```python
from build123d import *

# Parameters (mm, degrees)
SKETCH1_W           = 100
SKETCH1_H           = 100
BOSS_EXTRUDE1_DEPTH = 5.08
SKETCH2_R           = 40
BOSS_EXTRUDE2_DEPTH = 63.5
CHAMFER1_SIZE       = 5.08


with BuildPart() as part:
    # Sketch1 → Boss-Extrude1 (new body)
    with BuildSketch(Plane.XY):
        Rectangle(SKETCH1_W, SKETCH1_H)
    extrude(amount=BOSS_EXTRUDE1_DEPTH)

    # Sketch2 → Boss-Extrude2 (add)
    with BuildSketch(Plane.XY):
        Circle(SKETCH2_R)
    extrude(amount=BOSS_EXTRUDE2_DEPTH)

    # Chamfer1
    chamfer1_edges = [part.edges().sort_by_distance(p)[0] for p in [
        (-40, 0, 63.5),
    ]]
    chamfer(chamfer1_edges, length=CHAMFER1_SIZE)


solid = part.part
```
Could you check a few things on this model? Use its own coordinates, in mm. A direction names the side the tool comes from. Coordinates: 2 decimals unless noted, no trailing zeros. Loops run counter-clockwise (first coordinate to the right, second up) from the corner with the lowest first, then second, coordinate; pieces in that order, holes last.
1) Please list where these lines run through material, in increasing order: line 1 along Z through (x, y) = (41, -13); line 2 along X through (y, z) = (-16, 11.5); line 3 along X through (y, z) = (-18, 8).
Reported:
line 1: z = 0 to 5.08
line 2: x = -36.66 to 36.66
line 3: x = -35.72 to 35.72
2) Thinking about a two-plate mould opening in X: for faces 3 (the face through (33.543, 10.563, 63.253)), 4 (the face through (-1, -50, 3)), 5 (the face through (-50, -1, 3)), which applies, released by +X, released by -X, zero draft, split by the parting line, or undercut?
Reported:
face 3: split by the parting line
face 4: zero draft
face 5: released by -X
3) Imagine slicing it at C-C (z = 18.5). List the corners of the cut face in (x, y) for me, and give its area (3 significant figures).
Reported:
outline: circle Ø80 at (0, 0)
area: 5,030 mm2
4) Which directions (+Z, -Z, +X, -X, +Y, -Y) give clear straight access to the entire face, cutting with the end or side of a thin tool? Please do faces 1 (the face through (-1, 1, 0)), 2 (the face through (-34, 23, 5.08)).
Reported:
face 1: -Z, +X, -X, +Y, -Y
face 2: +Z
5) Imagine slicing it at A-A (y = 0). List the corners of the cut face in (x, z) for me, and give its area (3 significant figures).
Reported:
outline: (-50, 0) - (50, 0) - (50, 5.08) - (40, 5.08) - (40, 58.42) - (34.92, 63.5) - (-34.92, 63.5) - (-40, 58.42) - (-40, 5.08) - (-50, 5.08) - close
area: 5,160 mm2
6) Will these pins go through, and if not, where does the flat tip stop? pin 1 Ø3 at (x, z) = (-16, 40) entering from -Y; pin 2 Ø6 at (y, z) = (-21, 20) entering from -X; pin 3 Ø1 at (x, z) = (7, 50) entering from -Y.
Reported:
pin 1: stops at y = -37.28
pin 2: stops at x = -35.72
pin 3: stops at y = -39.47
